```python
from build123d import *

# Parameters (mm, degrees)
ENCLOSURE_SHELL_SKETCH_W      = 74
ENCLOSURE_SHELL_SKETCH_H      = 52
ENCLOSURE_SHELL_FEATURE_DEPTH = 32
ENCLOSURE_GAP_SKETCH_W        = 72
ENCLOSURE_GAP_SKETCH_H        = 50
ENCLOSURE_GAP_FEATURE_DEPTH   = 30
SCREW_SHELL_SKETCH_R          = 2.5
SCREW_SHELL_FEATURE_DEPTH     = 8
SCREW_HOLE_SKETCH_R           = 1.6
SCREW_HOLE_FEATURE_DEPTH      = 8
BATTERY_CUT_REACH             = 86.711
BATTERY_CUT_DIRECTION_2_DEPTH = 85.711274338
CAMERA_CORD_HOLE_SKETCH_W     = 8
CAMERA_CORD_HOLE_SKETCH_H     = 4
CAMERA_CORD_HOLE_DEPTH        = 55.267854205
TAB_FEATURE_SKETCH_W          = 8
TAB_FEATURE_SKETCH_H          = 5
TAB_FEATURE_DEPTH             = 15


with BuildPart() as part:
    # Enclosure Shell Sketch → Enclosure Shell Feature (new body)
    with BuildSketch(Plane(origin=(0, 0, 0), x_dir=(1, 0, 0), z_dir=(0, 1, 0))):
        Rectangle(ENCLOSURE_SHELL_SKETCH_W, ENCLOSURE_SHELL_SKETCH_H)
    extrude(amount=ENCLOSURE_SHELL_FEATURE_DEPTH)

    # Enclosure Gap Sketch → Enclosure Gap Feature (cut)
    with BuildSketch(Plane(origin=(0, 32, 0), x_dir=(1, 0, 0), z_dir=(0, 1, 0))):
        Rectangle(ENCLOSURE_GAP_SKETCH_W, ENCLOSURE_GAP_SKETCH_H)
    extrude(amount=-ENCLOSURE_GAP_FEATURE_DEPTH, mode=Mode.SUBTRACT)

    # Screw Shell Sketch → Screw Shell Feature (add)
    with BuildSketch(Plane(origin=(0, 2, 0), x_dir=(1, 0, 0), z_dir=(0, 1, 0))):
        with Locations(Location((-31.096, 20.5, 0), (0, 0, 270))):
            Circle(SCREW_SHELL_SKETCH_R)
        with Locations(Location((-31.096, -20.5, 0), (0, 0, 270))):
            Circle(SCREW_SHELL_SKETCH_R)
        with Locations(Location((31.1, 20.5, 0), (0, 0, 270))):
            Circle(SCREW_SHELL_SKETCH_R)
        with Locations(Location((31.1, -20.5, 0), (0, 0, 270))):
            Circle(SCREW_SHELL_SKETCH_R)
    extrude(amount=SCREW_SHELL_FEATURE_DEPTH)

    # Screw Hole Sketch → Screw Hole Feature (cut)
    with BuildSketch(Plane(origin=(0, 10, 0), x_dir=(1, 0, 0), z_dir=(0, 1, 0))):
        with Locations(Location((-31.096, 20.5, 0), (0, 0, 270))):
            Circle(SCREW_HOLE_SKETCH_R)
        with Locations(Location((-31.096, -20.5, 0), (0, 0, 270))):
            Circle(SCREW_HOLE_SKETCH_R)
        with Locations(Location((31.1, -20.5, 0), (0, 0, 270))):
            Circle(SCREW_HOLE_SKETCH_R)
        with Locations(Location((31.1, 20.5, 0), (0, 0, 270))):
            Circle(SCREW_HOLE_SKETCH_R)
    extrude(amount=-SCREW_HOLE_FEATURE_DEPTH, mode=Mode.SUBTRACT)

    # Battery Cut Sketch → Battery Cut (cut, up to next)
    with BuildSketch(Plane.ZY.offset(-37), mode=Mode.PRIVATE) as battery_cut_sk1:
        Polygon((0, 32), (7.492527579, 32), (7.492527579, 26), (-7.5, 26), (-7.5, 32), align=None)
    battery_cut_tool1 = extrude(battery_cut_sk1.sketch, amount=BATTERY_CUT_REACH, mode=Mode.PRIVATE) & part.part
    add(battery_cut_tool1.solids().sort_by_distance((37, 29, -0.003736))[0], mode=Mode.SUBTRACT)

    # Battery Cut Sketch → Battery Cut direction 2 (cut)
    with BuildSketch(Plane.ZY.offset(-37)):
        Polygon((0, 32), (7.492527579, 32), (7.492527579, 26), (-7.5, 26), (-7.5, 32), align=None)
    extrude(amount=-BATTERY_CUT_DIRECTION_2_DEPTH, mode=Mode.SUBTRACT)

    # Camera Cord Hole Sketch → Camera Cord Hole (cut, through all)
    with BuildSketch(Plane(origin=(0, 2, 0), x_dir=(1, 0, 0), z_dir=(0, 1, 0))):
        with Locations((-17, -13)):
            Rectangle(CAMERA_CORD_HOLE_SKETCH_W, CAMERA_CORD_HOLE_SKETCH_H)
    extrude(amount=-CAMERA_CORD_HOLE_DEPTH, mode=Mode.SUBTRACT)

    # Tab Feature Sketch → Tab Feature (add)
    with BuildSketch(Plane(origin=(0, 0, -26), x_dir=(-1, 0, 0), z_dir=(0, 0, -1))):
        with Locations((-29, 2.5)):
            Rectangle(TAB_FEATURE_SKETCH_W, TAB_FEATURE_SKETCH_H)
        with Locations((29, 2.5)):
            Rectangle(TAB_FEATURE_SKETCH_W, TAB_FEATURE_SKETCH_H)
    extrude(amount=TAB_FEATURE_DEPTH)


solid = part.part
```
Source: CAD feature listing. Evaluate the final solid. Frame: model axes, mm. A direction names the side the tool comes from. Round coordinates to 2 decimals unless told otherwise and drop trailing zeros. Write each loop counter-clockwise with the first axis right and the second up, starting at its lowest first coordinate (ties: lowest second). Pieces come first, ordered by that corner, then holes. Notation, with made-up numbers: M -31,16 L -13,16 A13 cw -13,25 Z; hole C 22,-24 d6. An arc over 180 degrees is marked long. Use CSV: the item, a comma, the result in double quotes. Start each with the question number.
Q1. Access query for faces 1 (the face through (-21, 1, 13)), 2 (the face through (-31, 2, -21)), 3 (the face through (-33, 2, -33)), 4 (the face through (-29, 5, -33)), 5 (the face through (33, 2, -33)). Directions: +Z, -Z, +X, -X, +Y, -Y. A direction counts if a zero-diameter tool reaches every point of the face in a straight line with its end or side. Return the directions, or none.
Q2. Cut plane D-D on z = 20.5. Output: boundary loops of the cut face in (x, y).
Q3. First-contact query: P1, Ø25, axis at x = -9.5, z = 8.5, coming from the +Y side; P2, Ø12, axis at x = 3, y = 18.5, coming from the -Z side; P3, Ø2.5, axis at x = 31.5, z = 20, coming from the +Y side. Flat tips, straight axial feed; report the tip coordinate or a pass-through.
Q4. Pull-direction query (Z, two-part tool) for faces 6 (the face through (29, 3, -41)), 7 (the face through (29.6, 5.9, -22.5)), 8 (the face through (25, 2, -33)); classes: +Z half, -Z half, draft (parallel to the pull), parting line (faces both ways), or undercut.
Q5. Cut plane C-C on y = 19.5. Output: boundary loops of the cut face in (x, z).
Q6. Cut plane A-A on z = 12.5. Output: boundary loops of the cut face in (x, y).
Q7. Line query: line 1 (X direction, y = 6.5, z = -20.5); line 2 (X direction, y = 23.5, z = 11); line 3 (X direction, y = 4, z = -27.5). Output: solid intervals per line, ascending. Write a range as from..to.
Q8. Cut plane B-B on y = 29. Output: boundary loops of the cut face in (x, z), plus the area to 3 significant figures.
Results found:
1,face 1,"+Y, -Y"
1,face 2,"+Y"
1,face 3,"-Z, -X, +Y, -Y"
1,face 4,"-Z, +X, -X, +Y"
1,face 5,"-Z, +X, +Y, -Y"
2,outline,"M -37,0 L 37,0 L 37,32 L 36,32 L 36,2 L 33.6,2 L 33.6,10 L 32.7,10 L 32.7,2 L 29.5,2 L 29.5,10 L 28.6,10 L 28.6,2 L -28.6,2 L -28.6,10 L -29.5,10 L -29.5,2 L -32.7,2 L -32.7,10 L -33.6,10 L -33.6,2 L -36,2 L -36,32 L -37,32 Z"
3,P1,"y = 2"
3,P2,"z = -26"
3,P3,"y = 10"
4,face 6,"-Z half"
4,face 7,"undercut"
4,face 8,"draft"
5,outline,"M -37,-26 L 37,-26 L 37,26 L -37,26 Z; hole M -36,-25 L 36,-25 L 36,25 L -36,25 Z"
6,outline,"M -37,0 L -21,0 L -21,2 L -36,2 L -36,32 L -37,32 Z; M -13,0 L 37,0 L 37,32 L 36,32 L 36,2 L -13,2 Z"
7,line 1,"-37..-36, -33.6..-32.7, -29.5..-28.6, 28.6..29.5, 32.7..33.6, 36..37"
7,line 2,"-37..-36, 36..37"
7,line 3,"-33..-25, 25..33"
8,outline,"M -37,-26 L 37,-26 L 37,-7.5 L 36,-7.5 L 36,-25 L -36,-25 L -36,25 L 36,25 L 36,7.49 L 37,7.49 L 37,26 L -37,26 Z"
8,area,"233 mm^2"
